Autodesk Inventor part; units mm, degrees
ref_plane "YZ Plane" through (0, 0, 0) normal (1, 0, 0) x (0, 1, 0)
ref_plane "XZ Plane" through (0, 0, 0) normal (0, 1, 0) x (-1, 0, 0)
ref_plane "XY Plane" through (0, 0, 0) normal (0, 0, 1) x (1, 0, 0)
sketch "スケッチ1" plane through (0, 0, 0) normal (0, 1, 0) x (-1, 0, 0)
  line L0 (0, 0) -> (15, 0)
  line L1 (15, 0) -> (15, -15)
  line L2 (15, -15) -> (0, -15)
  line L3 (0, -15) -> (0, 0)
  dimension "d0" = 15
  dimension "d1" = 15
extrude "押し出し1" add sketch "スケッチ1" along normal blind 100
sketch "スケッチ2" plane through (0, 100, 0) normal (0, 1, 0) x (1, 0, 0)
  line L0 (-13.5, 13.5) -> (-1.5, 13.5)
  line L1 (-1.5, 13.5) -> (-1.5, 1.5)
  line L2 (-1.5, 1.5) -> (-13.5, 1.5)
  line L3 (-13.5, 1.5) -> (-13.5, 13.5)
  line L4 (-15, 15) -> (-15, 0)
  line L5 (0, 15) -> (-15, 15)
  point P0 (0, 0)
  dimension "d4" = 12
  dimension "d5" = 12
  dimension "d6" = 1.5
  dimension "d7" = 1.5
extrude "押し出し2" cut sketch "スケッチ2" against normal blind 100
sketch "スケッチ3" plane through (0, 0, 0) normal (1, 0, 0) x (0, 0, -1)
  point P0 (0, 0)
sketch "スケッチ4" plane through (0, 0, 0) normal (1, 0, 0) x (0, 0, -1)
  line L0 (0, 100) -> (15, 100)
  line L1 (0, 0) -> (0, 100)
  point P0 (7.5, 90)
  point P1 (7.5, 80)
  dimension "d10" = 10
  dimension "d11" = 7.5
  dimension "d12" = 10
  dimension "d13" = 7.5
hole "穴1" at (0, 90, -7.5) at (0, 80, -7.5) direction (-1, 0, 0) diameter 3.2 end through all
Work out the finished part from the listing and answer in its coordinate system (mm). A direction names the side the tool comes from. Round coordinates to 2 decimals unless told otherwise and drop trailing zeros. Write each loop counter-clockwise with the first axis right and the second up, starting at its lowest first coordinate (ties: lowest second). Pieces come first, ordered by that corner, then holes. Notation, with made-up numbers: (-34.75, 55.5) - (-12.75, 55.5) arc R32 cw to (-12.75, 83.5) - close; hole circle Ø9 at (52, 9.5). An arc over 180 degrees is marked (long way). Return JSON: item names as keys, results as strings. Group by question number.
Q1. For faces 1 (the flat face through (-13.5, 51, -7)), 2 (the flat face through (0, 49, -8)), determine the directions among +Z, -Z, +X, -X, +Y, -Y from which every point of the face is accessible in a straight line to the end or side of a thin tool.
Q2. The part is cut by section D-D on y = 63.5. Write down the section's boundary in (x, z).
Q3. The part is cut by section B-B on z = -7.5. Write down the section's boundary in (x, y).
Q4. The mould has two halves that part along Y. Classify faces 3 (the flat face through (-14, 0, -7)), 4 (the flat face through (-14, 100, -7)), 5 (the cylindrical face through (-14.26, 78.414, -7.292)), 6 (the flat face through (-8, 51, -13.5)): released by +Y, released by -Y, zero draft, split by the parting line, or undercut.
Q5. Find the intervals of material crossed by L1, parallel to Y at x = -14, z = -7.5; L2, parallel to X at y = 27.5, z = -1.75; L3, parallel to Z at x = -14.3, y = 90, in increasing order.
Q6. The part is cut by section A-A on x = -3.5. Write down the section's boundary in (y, z), then the cut area to 3 significant figures.
Q7. The part is cut by section C-C on y = 80. Write down the section's boundary in (x, z), then the cut area to 3 significant figures.
Solved:
{
 "1": {"face 1": "+Y, -Y", "face 2": "+Z, -Z, +X, +Y, -Y"},
 "2": {"outline": "(-15, -15) - (0, -15) - (0, 0) - (-15, 0) - close; hole (-13.5, -13.5) - (-1.5, -13.5) - (-1.5, -1.5) - (-13.5, -1.5) - close"},
 "3": {"outline": "(-15, 0) - (-13.5, 0) - (-13.5, 78.4) - (-15, 78.4) - close; (-15, 81.6) - (-13.5, 81.6) - (-13.5, 88.4) - (-15, 88.4) - close; (-15, 91.6) - (-13.5, 91.6) - (-13.5, 100) - (-15, 100) - close; (-1.5, 0) - (0, 0) - (0, 78.4) - (-1.5, 78.4) - close; (-1.5, 81.6) - (0, 81.6) - (0, 88.4) - (-1.5, 88.4) - close; (-1.5, 91.6) - (0, 91.6) - (0, 100) - (-1.5, 100) - close"},
 "4": {"face 3": "released by -Y", "face 4": "released by +Y", "face 5": "undercut", "face 6": "zero draft"},
 "5": {"L1": "0 to 78.4, 81.6 to 88.4, 91.6 to 100", "L2": "-15 to -13.5, -1.5 to 0", "L3": "-15 to -9.1, -5.9 to 0"},
 "6": {"outline": "(0, -15) - (100, -15) - (100, -13.5) - (0, -13.5) - close; (0, -1.5) - (100, -1.5) - (100, 0) - (0, 0) - close", "area": "300 mm²"},
 "7": {"outline": "(-15, -15) - (0, -15) - (0, -9.1) - (-1.5, -9.1) - (-1.5, -13.5) - (-13.5, -13.5) - (-13.5, -9.1) - (-15, -9.1) - close; (-15, -5.9) - (-13.5, -5.9) - (-13.5, -1.5) - (-1.5, -1.5) - (-1.5, -5.9) - (0, -5.9) - (0, 0) - (-15, 0) - close", "area": "71.4 mm²"}
}
